For this review, take the finished solid that the model builds, in its own axes (mm). Give positions to 0.01 mm unless a question says otherwise; leave off trailing zeros. Order: outer loops, then holes, each group sorted by start corner. A loop starts at its lowest first (then second) coordinate and runs counter-clockwise, first axis right, second up.
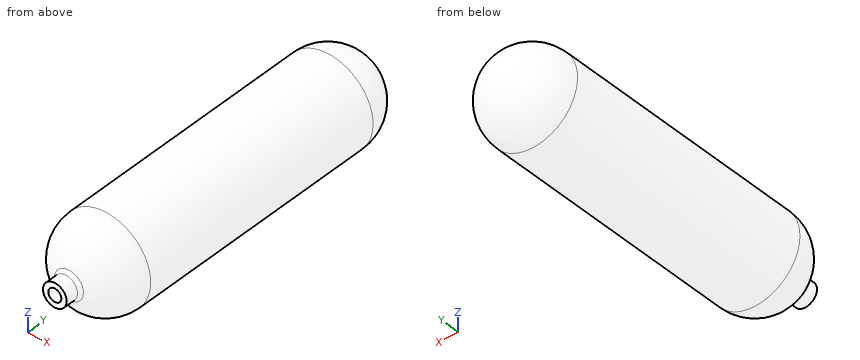
from build123d import *

# Parameters (mm, degrees)
M18X1_5_TAPPED_HOLE1_D     = 16.5
M18X1_5_TAPPED_HOLE1_DEPTH = 15.042899893
M18X1_5_TAPPED_HOLE1_TIP   = 4.957100107
FILLET1_R                  = 5


with BuildPart() as part:
    # Sketch1 → Revolve1 (revolve)
    with BuildSketch(Plane.XY, mode=Mode.PRIVATE) as revolve1_sk:
        with BuildLine():
            Line((0, 0), (15, 0))
            Line((15, 0), (15, 20))
            ThreePointArc((15, 20), (45.654955919, 40.553679643), (57.5, 75.509008278))
            Line((57.5, 75.509008278), (57.5, 407.5))
            ThreePointArc((57.5, 407.5), (40.658639918, 448.158639918), (0, 465))
            Line((0, 465), (0, 0))
        make_face()
    revolve(revolve1_sk.sketch.rotate(Axis((0, 0, 0), (0, 1, 0)), 90), axis=Axis((0, 0, 0), (0, 1, 0)))

    # M18x1.5 Tapped Hole1
    with Locations(Plane(origin=(0, 0, 0), x_dir=(-1, 0, 0), z_dir=(0, -1, 0))):
        with Locations((0, 0)):
            Hole(M18X1_5_TAPPED_HOLE1_D / 2, depth=M18X1_5_TAPPED_HOLE1_DEPTH)
            with Locations((0, 0, -(M18X1_5_TAPPED_HOLE1_DEPTH + M18X1_5_TAPPED_HOLE1_TIP / 2))):  # 118° drill point
                Cone(0, M18X1_5_TAPPED_HOLE1_D / 2, M18X1_5_TAPPED_HOLE1_TIP, mode=Mode.SUBTRACT)

    # Fillet1
    fillet1_edges = [part.edges().sort_by_distance(p)[0] for p in [
        (0, 20, 15),
    ]]
    fillet(fillet1_edges, radius=FILLET1_R)

    # Sketch4 → Cut-Revolve1 (revolve, cut)
    with BuildSketch(Plane.XY):
        with BuildLine():
            Line((8.25, 15.042899893), (8.25, 25.769587292))
            Line((8.25, 25.769587292), (16.8, 25.769587292))
            ThreePointArc((16.8, 25.769587292), (42.651201624, 44.89651083), (52.5, 75.509008278))
            Line((52.5, 75.509008278), (52.5, 407.5))
            ThreePointArc((52.5, 407.5), (37.123106012, 444.623106012), (0, 460))
            Line((0, 460), (0, 15.042899893))
            Line((0, 15.042899893), (8.25, 15.042899893))
        make_face()
    revolve(axis=Axis((0, 0, 0), (0, 1, 0)), mode=Mode.SUBTRACT)


solid = part.part
1) To check wall thickness, follow line 1 (X direction, y = 5, z = 0); line 2 (X direction, y = 160, z = 0); line 3 (Z direction, x = 2, y = 296). State the ranges of each line that lie inside material, in increasing order.
Answer sheet:
line 1: x = -15 to -8.25, 8.25 to 15
line 2: x = -57.5 to -52.5, 52.5 to 57.5
line 3: z = -57.47 to -52.46, 52.46 to 57.47
2) We need section A-A on z = -24.5. Give the boundary of the cut face in (x, y).
Answer sheet:
outline: (-52.02, 75.51) arc R52.02 ccw to (52.02, 75.51) - (52.02, 407.5) arc R52.02 ccw to (-52.02, 407.5) - close; hole (-46.43, 75.51) arc R46.43 ccw to (46.43, 75.51) - (46.43, 407.5) arc R46.43 ccw to (-46.43, 407.5) - close
3) We need section B-B on x = -48. Give the boundary of the cut face in (y, z).
Answer sheet:
outline: (75.51, -31.66) - (407.5, -31.66) arc R31.66 ccw to (407.5, 31.66) - (75.51, 31.66) arc R31.66 ccw to start; hole (75.51, -21.27) - (407.5, -21.27) arc R21.27 ccw to (407.5, 21.27) - (75.51, 21.27) arc R21.27 ccw to start
4) Clearance check with flat-ended pins moving along their axes: pin 1 (4 mm diameter, centred on x = -26, y = 177, fed in from +Z); pin 2 (3 mm diameter, centred on y = 54, z = -16, fed in from +X); pin 3 (5 mm diameter, centred on x = 24.5, z = 12, fed in from -Y). State where each tip first meets the part, or that it passes through.
Answer sheet:
pin 1: stops at z = 52.25
pin 2: stops at x = 51.63
pin 3: stops at y = 23.62
5) We need section C-C on y = 137. Give the boundary of the cut face in (x, z).
Answer sheet:
outline: circle Ø115 at (0, 0); hole circle Ø105 at (0, 0)
